Verification items for the finished model (mm, model axes). A direction names the side the tool comes from. Coordinates: 2 decimals unless noted, no trailing zeros. Write each loop counter-clockwise with the first axis right and the second up, starting at its lowest first coordinate (ties: lowest second). Pieces come first, ordered by that corner, then holes. Notation, with made-up numbers: (30, -4.5) -> (85, -4.5) arc R17 cw to (85, 26.5) -> close; hole circle Ø11 at (-32.5, 83.25). An arc over 180 degrees is marked (long way). Answer in a Markdown table with one row per item.
```python
from build123d import *

# Parameters (mm, degrees)
F3_DEPTH = 15
F2_W     = 1.932107
F2_H     = 6
F4_DEPTH = 4
F5_R     = 0.7
F6_R     = 0.7


with BuildPart() as f1:
    # F0 (on Front) → F1 (revolve)
    with BuildSketch(Plane.XZ):
        with BuildLine():
            Line((-2, 20), (-30, 20))
            Line((-30, 20), (-29.773503, 3.94358))
            ThreePointArc((-29.773503, 3.94358), (-28.58231, 1.151695), (-25.773901, 0))
            Line((-25.773901, 0), (-4.717873, 0))
            Line((-4.717873, 0), (-4.717873, 16))
            Line((-4.717873, 16), (-2, 16))
            Line((-2, 16), (-2, 20))
        make_face()
    revolve(axis=Axis((0, 0, 6.694083), (0, 0, -1)))

    # F2 (on face) → F3 (cut)
    with BuildSketch(Plane.XY.offset(20)):
        with BuildLine():
            Line((-1, -25.842809), (-1, -8.251002))
            ThreePointArc((-1, -8.251002), (-5.877033, -5.877033), (-8.251002, -1))
            Line((-8.251002, -1), (-25.842809, -1))
            ThreePointArc((-25.842809, -1), (-18.287302, -18.287302), (-1, -25.842809))
        make_face()
        with BuildLine():
            ThreePointArc((8.183109, -1.025774), (5.80914, -5.902807), (0.932107, -8.276776))
            Line((0.932107, -8.276776), (0.932107, -25.868583))
            ThreePointArc((0.932107, -25.868583), (18.219408, -18.313075), (25.774916, -1.025774))
            Line((25.774916, -1.025774), (8.183109, -1.025774))
        make_face()
        with BuildLine():
            ThreePointArc((0.957881, 8.157335), (5.834914, 5.783366), (8.208883, 0.906333))
            Line((8.208883, 0.906333), (25.80069, 0.906333))
            ThreePointArc((25.80069, 0.906333), (18.245182, 18.193635), (0.957881, 25.749142))
            Line((0.957881, 25.749142), (0.957881, 23))
            Line((0.957881, 23), (0.957881, 17))
            Line((0.957881, 17), (0.957881, 8.157335))
        make_face()
        with BuildLine():
            Line((-0.974226, 8.183109), (-0.974226, 17))
            Line((-0.974226, 17), (-0.974226, 23))
            Line((-0.974226, 23), (-0.974226, 25.774916))
            ThreePointArc((-0.974226, 25.774916), (-18.261528, 18.219408), (-25.817035, 0.932107))
            Line((-25.817035, 0.932107), (-8.225228, 0.932107))
            ThreePointArc((-8.225228, 0.932107), (-5.851259, 5.80914), (-0.974226, 8.183109))
        make_face()
    extrude(amount=-F3_DEPTH, mode=Mode.SUBTRACT)

    # F2 (on face) → F4 (join)
    with BuildSketch(Plane.XY.offset(20)):
        with Locations((-0.008172, 20)):
            Rectangle(F2_W, F2_H)
    extrude(amount=F4_DEPTH)

    # F5
    f5_edges = [f1.edges().sort_by_distance(p)[0] for p in [
        (-0.974226, 20, 24),
    ]]
    fillet(f5_edges, radius=F5_R)

    # F6
    f6_edges = [f1.edges().sort_by_distance(p)[0] for p in [
        (0.957881, 20, 24),
    ]]
    fillet(f6_edges, radius=F6_R)


solid = f1.part
```
1. Sectioned sample at C-C, the plane z = 6.5. Record the cut outline in (x, y), and give its area (3 significant figures).
Findings below:
| item | result |
|---|---|
| outline | circle Ø59.62 at (0, 0); hole (-25.84, -1) arc R25.86 ccw to (-1, -25.84) -> (-1, -8.25) arc R8.31 cw to (-8.25, -1) -> close; hole (-25.82, 0.93) -> (-8.23, 0.93) arc R8.31 cw to (-0.97, 8.18) -> (-0.97, 25.77) arc R25.86 ccw to start; hole circle Ø9.44 at (0, 0); hole (0.93, -25.87) arc R25.86 ccw to (25.77, -1.03) -> (8.18, -1.03) arc R8.31 cw to (0.93, -8.28) -> close; hole (0.96, 8.16) arc R8.31 cw to (8.21, 0.91) -> (25.8, 0.91) arc R25.86 ccw to (0.96, 25.75) -> close |
| area | 978 mm² |
2. Material ranges on probe 1 along Y at (x, z) = (-15, 15.75); probe 2 along Y at (x, z) = (0, 3.75); probe 3 along X at (y, z) = (8.5, 14.25), recorded low to high. Write a range as from..to.
Findings below:
| item | result |
|---|---|
| probe 1 | y = -25.91..-21.07, -1..0.93, 20.98..25.91 |
| probe 2 | y = -29.77..-4.72, 4.72..29.77 |
| probe 3 | x = -28.69..-24.38, -0.97..0.96, 24.35..28.69 |
3. Sectioned sample at B-B, the plane z = 21.75. Record the cut outline in (x, y).
Findings below:
| item | result |
|---|---|
| outline | (-0.97, 17) -> (0.96, 17) -> (0.96, 23) -> (-0.97, 23) -> close |
4. Go/stop test with flat-tipped pins: pin 1 (1.7 mm diameter, centred on y = 19.5, z = 21.5, fed in from +X); pin 2 (1 mm diameter, centred on y = 16.5, z = 18.5, fed in from +X); pin 3 (3.5 mm diameter, centred on y = 19, z = 22.5, fed in from -X). Record where each tip stops, or that it passes through.
Findings below:
| item | result |
|---|---|
| pin 1 | stops at x = 0.96 |
| pin 2 | stops at x = 25.35 |
| pin 3 | stops at x = -0.97 |
5. Sectioned sample at A-A, the plane z = 17.25. Record the cut outline in (x, y).
Findings below:
| item | result |
|---|---|
| outline | circle Ø59.92 at (0, 0); hole (-25.84, -1) arc R25.86 ccw to (-1, -25.84) -> (-1, -8.25) arc R8.31 cw to (-8.25, -1) -> close; hole (-25.82, 0.93) -> (-8.23, 0.93) arc R8.31 cw to (-0.97, 8.18) -> (-0.97, 25.77) arc R25.86 ccw to start; hole circle Ø4 at (0, 0); hole (0.93, -25.87) arc R25.86 ccw to (25.77, -1.03) -> (8.18, -1.03) arc R8.31 cw to (0.93, -8.28) -> close; hole (0.96, 8.16) arc R8.31 cw to (8.21, 0.91) -> (25.8, 0.91) arc R25.86 ccw to (0.96, 25.75) -> close |
6. Access from +Z, -Z, +X, -X, +Y, -Y to the whole of each face (thin tool, end or side, straight path). Record for faces 4 (the face through (1.023, -4.606, 8.112)), 5 (the face through (-0.974, 20, 22)), 6 (the face through (5.86, -5.85, 12.6)).
Findings below:
| item | result |
|---|---|
| face 4 | -Z |
| face 5 | +Z, -X, +Y, -Y |
| face 6 | +Z |
7. Release check for a two-part mould opening along X. For faces 1 (the face through (0.958, 20, 22)), 2 (the face through (0, -6, 20)), 3 (the face through (-17, 0.932, 13)) record: released by +X, released by -X, zero draft, split by the parting line, or undercut.
Findings below:
| item | result |
|---|---|
| face 1 | released by +X |
| face 2 | zero draft |
| face 3 | undercut |
